from build123d import *

# Parameters (mm, degrees)
F0_W        = 88.9
F0_H        = 88.9
F1_DEPTH    = 19.05
F3_DEPTH    = 12.7
F4_T1_DEPTH = 209.55
F5_W        = 3.81
F5_H        = 5.08
F6_DEPTH    = 38.1
F7_W        = 3.81
F7_H        = 5.08
F8_DEPTH    = 38.1
F9_W        = 3.81
F9_H        = 5.08
F10_DEPTH   = 38.1
F11_W       = 3.81
F11_H       = 5.08
F12_DEPTH   = 38.1
F13_W       = 3.81
F13_H       = 5.08
F14_DEPTH   = 38.1
F15_W       = 3.81
F15_H       = 5.08
F16_DEPTH   = 38.1
F17_W       = 3.81
F17_H       = 5.08
F18_DEPTH   = 38.1
F19_W       = 3.81
F19_H       = 5.08
F20_DEPTH   = 38.1


# Not quite as in the source:
# - a fillet or chamfer that OpenCascade refuses, or shapes differently, is made with other operations: its cross-section is extruded or revolved along the edge and cut away or added


with BuildPart() as f1:
    # F0 (on Top) → F1 (new body)
    with BuildSketch(Plane.XY):
        with Locations((44.45, 44.45)):
            Rectangle(F0_W, F0_H)
    extrude(amount=F1_DEPTH)

    # F2 (on face) → F3 (cut)
    with BuildSketch(Plane.XY.offset(19.05)):
        Polygon((38.1, 50.8), (0, 50.8), (0, 38.1), (38.1, 38.1), (38.1, 0), (50.8, 0), (50.8, 38.1), (88.9, 38.1), (88.9, 50.8), (50.8, 50.8), (50.8, 88.9), (38.1, 88.9), align=None)
    extrude(amount=-F3_DEPTH, mode=Mode.SUBTRACT)

    # F4: fillet of radius 38.1 on 4 edges, made by hand

    # F4_s2 → F4_t1 (cut)
    with BuildSketch(Plane.XY.offset(-95.25)):
        with BuildLine():
            ThreePointArc((50.8, 0), (77.7407683632, 11.1592316368), (88.9, 38.1))
            Line((88.9, 38.1), (88.9, 0))
            Line((88.9, 0), (50.8, 0))
        make_face()
        with BuildLine():
            ThreePointArc((0, 38.1), (11.1592316368, 11.1592316368), (38.1, 0))
            Line((38.1, 0), (0, 0))
            Line((0, 0), (0, 38.1))
        make_face()
        with BuildLine():
            ThreePointArc((50.8, 88.9), (77.7407683632, 77.7407683632), (88.9, 50.8))
            Line((88.9, 50.8), (88.9, 88.9))
            Line((88.9, 88.9), (50.8, 88.9))
        make_face()
        with BuildLine():
            ThreePointArc((0, 50.8), (11.1592316368, 77.7407683632), (38.1, 88.9))
            Line((38.1, 88.9), (0, 88.9))
            Line((0, 88.9), (0, 50.8))
        make_face()
    extrude(amount=F4_T1_DEPTH, mode=Mode.SUBTRACT)

    # F5 (on face) → F6 (cut)
    with BuildSketch(Plane(origin=(0, 38.1, 0), x_dir=(-1, 0, 0), z_dir=(0, 1, 0))):
        with Locations((-52.705, 12.7)):
            Rectangle(F5_W, F5_H)
    extrude(amount=-F6_DEPTH, mode=Mode.SUBTRACT)

    # F7 (on face) → F8 (cut)
    with BuildSketch(Plane.XZ.offset(-50.8)):
        with Locations((52.705, 12.7)):
            Rectangle(F7_W, F7_H)
    extrude(amount=-F8_DEPTH, mode=Mode.SUBTRACT)

    # F9 (on face) → F10 (cut)
    with BuildSketch(Plane.YZ.offset(38.1)):
        with Locations((36.195, 12.7)):
            Rectangle(F9_W, F9_H)
    extrude(amount=-F10_DEPTH, mode=Mode.SUBTRACT)

    # F11 (on face) → F12 (cut)
    with BuildSketch(Plane(origin=(54.61, 0, 0), x_dir=(0, -1, 0), z_dir=(-1, 0, 0))):
        with Locations((-36.195, 12.7)):
            Rectangle(F11_W, F11_H)
    extrude(amount=-F12_DEPTH, mode=Mode.SUBTRACT)

    # F13 (on face) → F14 (cut)
    with BuildSketch(Plane.YZ.offset(38.1)):
        with Locations((52.705, 12.7)):
            Rectangle(F13_W, F13_H)
    extrude(amount=-F14_DEPTH, mode=Mode.SUBTRACT)

    # F15 (on face) → F16 (cut)
    with BuildSketch(Plane(origin=(54.61, 0, 0), x_dir=(0, -1, 0), z_dir=(-1, 0, 0))):
        with Locations((-52.705, 12.7)):
            Rectangle(F15_W, F15_H)
    extrude(amount=-F16_DEPTH, mode=Mode.SUBTRACT)

    # F17 (on face) → F18 (cut)
    with BuildSketch(Plane.XZ.offset(-54.61)):
        with Locations((36.195, 12.7)):
            Rectangle(F17_W, F17_H)
    extrude(amount=-F18_DEPTH, mode=Mode.SUBTRACT)

    # F19 (on face) → F20 (cut)
    with BuildSketch(Plane(origin=(0, 34.29, 0), x_dir=(-1, 0, 0), z_dir=(0, 1, 0))):
        with Locations((-36.195, 12.7)):
            Rectangle(F19_W, F19_H)
    extrude(amount=-F20_DEPTH, mode=Mode.SUBTRACT)


solid = f1.part
Verification items for the finished model (mm, model axes). A direction names the side the tool comes from. Coordinates: 2 decimals unless noted, no trailing zeros. Order: outer loops, then holes, each group sorted by start corner. A loop starts at its lowest first (then second) coordinate and runs counter-clockwise, first axis right, second up. Notation, with made-up numbers: (13, 7) -> (30, 7) arc R9 ccw to (30, 11) -> close; hole circle Ø5 at (72.5, 68). An arc over 180 degrees is marked (long way). Use CSV: the item, a comma, the result in double quotes. Start each with the question number.
Q1. Section check C-C, the plane z = 2.25. Record the cut outline in (x, y), and give its area (3 significant figures).
Q2. Depth check by flat-ended pin: P1, Ø1.5, axis at x = 51, z = 10.5, coming from the -Y side; P2, Ø1.9, axis at y = 74.5, z = 8.5, coming from the +X side; P3, Ø4, axis at x = 48.5, y = 10.5, coming from the +Z side; P4, Ø4, axis at x = 65, z = 11.5, coming from the +Y side. Enter the tip coordinate at first touch or a pass-through.
Q3. Section check B-B, the plane x = 52. Record the cut outline in (y, z).
Q4. Tool access check on faces 1 (the flat face through (35, 26, 10.16)), 2 (the flat face through (50.8, 70, 17)), 3 (the flat face through (19, 38.1, 8)). Record the directions out of +Z, -Z, +X, -X, +Y, -Y that give a thin tool (end or side, any length) a straight path to the whole face; none if there is none.
Q5. Section check A-A, the plane z = 14. Record the cut outline in (x, y).
Q6. Thickness scan on line 1 along Z through (x, y) = (53, 21); line 2 along X through (y, z) = (56, 9); line 3 along Z through (x, y) = (38.5, 28). Record the ranges inside material, lowest first.
Q7. Draft check along Z on faces 4 (the flat face through (54.61, 17, 13)), 5 (the flat face through (19, 50.8, 8)), 6 (the flat face through (54.61, 71, 13)), 7 (the flat face through (23, 66, 19.05)). Enter one of: +Z half, -Z half, draft (parallel to the pull), parting line (faces both ways), or undercut.
Q8. Section check D-D, the plane y = 21. Record the cut outline in (x, z), and give its area (3 significant figures).
Returned:
1,outline,"(0, 38.1) arc R38.1 ccw to (38.1, 0) -> (50.8, 0) arc R38.1 ccw to (88.9, 38.1) -> (88.9, 50.8) arc R38.1 ccw to (50.8, 88.9) -> (38.1, 88.9) arc R38.1 ccw to (0, 50.8) -> close"
1,area,"6,660 mm^2"
2,P1,"stops at y = 0"
2,P2,"stops at x = 81.36"
2,P3,"stops at z = 6.35"
2,P4,"stops at y = 86.89"
3,outline,"(0.02, 0) -> (88.88, 0) -> (88.88, 10.16) -> (50.8, 10.16) -> (50.8, 6.35) -> (38.1, 6.35) -> (38.1, 10.16) -> (0.02, 10.16) -> close; (0.02, 15.24) -> (38.1, 15.24) -> (38.1, 19.05) -> (0.02, 19.05) -> close; (50.8, 15.24) -> (88.88, 15.24) -> (88.88, 19.05) -> (50.8, 19.05) -> close"
4,face 1,"none"
4,face 2,"+Z, +Y, -Y"
4,face 3,"+Z, +X, -X"
5,outline,"(0.19, 34.29) arc R38.1 ccw to (34.29, 0.19) -> (34.29, 34.29) -> close; (0.19, 54.61) -> (34.29, 54.61) -> (34.29, 88.71) arc R38.1 ccw to start; (54.61, 0.19) arc R38.1 ccw to (88.71, 34.29) -> (54.61, 34.29) -> close; (54.61, 54.61) -> (88.71, 54.61) arc R38.1 ccw to (54.61, 88.71) -> close"
6,line 1,"z = 0 to 10.16, 15.24 to 19.05"
6,line 2,"x = 0.36 to 38.1, 50.8 to 88.54"
6,line 3,"z = 0 to 6.35"
7,face 4,"undercut"
7,face 5,"draft"
7,face 6,"undercut"
7,face 7,"+Z half"
8,outline,"(4.05, 0) -> (84.85, 0) -> (84.85, 19.05) -> (50.8, 19.05) -> (50.8, 15.24) -> (54.61, 15.24) -> (54.61, 10.16) -> (50.8, 10.16) -> (50.8, 6.35) -> (38.1, 6.35) -> (38.1, 10.16) -> (34.29, 10.16) -> (34.29, 15.24) -> (38.1, 15.24) -> (38.1, 19.05) -> (4.05, 19.05) -> close"
8,area,"1,340 mm^2"
